Could you check a few things on this drawing? It's one solid part, dimensions in mm from its lowest x, y, z. Round coordinates to 2 decimals unless told otherwise and drop trailing zeros. Write each loop counter-clockwise with the first axis right and the second up, starting at its lowest first coordinate (ties: lowest second). Pieces come first, ordered by that corner, then holes. Notation, with made-up numbers: M 66.25,-7 L 82.25,-7 A31 cw 82.25,26 Z; hole C 73.5,-17 d3. An arc over 180 degrees is marked long. One line per item, written item: value. Start each with the question number.
(1) Thinking about a two-plate mould opening in Z: for the marked faces 1 and 2, which applies, released by +Z, released by -Z, zero draft, split by the parting line, or undercut?
(2) I'm going to push flat-ended pins straight in: pin 1 Ø1.5 at (x, y) = (29, 93.5) entering from +Z; pin 2 Ø4 at (x, y) = (27.5, 81) entering from +Z. Where does each tip first touch, or does it pass through?
(3) I want a section at B-B on z = 283. Please give me the cut outline in (x, y) (1 decimal).
(4) If I drill on L1, parallel to Z at x = 67, y = 118; L2, parallel to Z at x = 69, y = 86; L3, parallel to Z at x = 88.5, y = 99, over which ranges is the centre line in solid material (lowest first)?
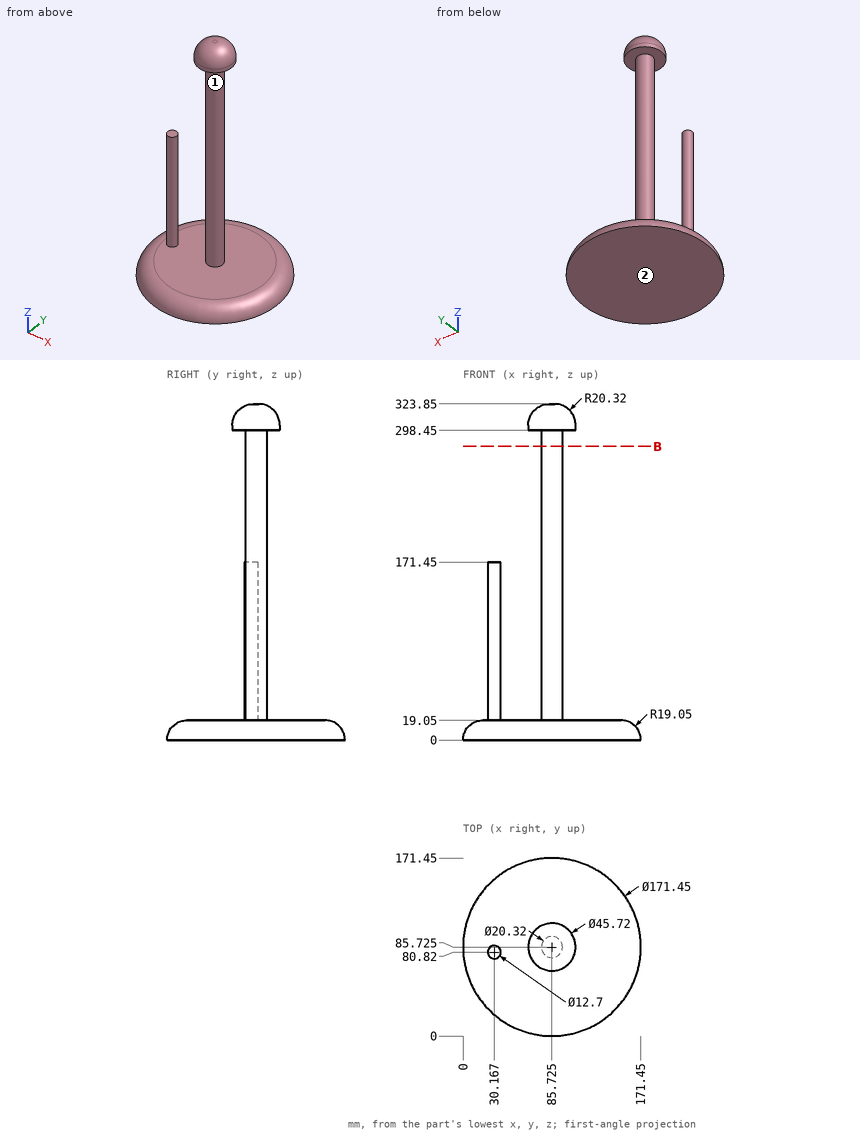
Found:
1. face 1: undercut
1. face 2: released by -Z
2. pin 1: stops at z = 19.05
2. pin 2: stops at z = 171.45
3. outline: C 85.7,85.7 d20.3
4. L1: z = 0 to 19.05
4. L2: z = 0 to 19.05, 298.45 to 318.08
4. L3: z = 0 to 19.05, 298.45 to 320.6
